from build123d import *

# Parameters (mm, degrees)
SKETCH1_W           = 9
SKETCH1_H           = 10
BOSS_EXTRUDE1_DEPTH = 3
SKETCH2_W           = 3
SKETCH2_H           = 10
BOSS_EXTRUDE2_DEPTH = 9
SKETCH3_W           = 10
SKETCH3_H           = 3
BOSS_EXTRUDE3_DEPTH = 17
SKETCH4_W           = 3
SKETCH4_H           = 10
BOSS_EXTRUDE4_DEPTH = 10
SKETCH5_W           = 10
SKETCH5_H           = 3
BOSS_EXTRUDE5_DEPTH = 6
CUT_EXTRUDE1_DEPTH  = 6


with BuildPart() as part:
    # Sketch1 → Boss-Extrude1 (new body)
    with BuildSketch(Plane(origin=(0, 0, 0), x_dir=(1, 0, 0), z_dir=(0, 1, 0))):
        with Locations((4.5, 5)):
            Rectangle(SKETCH1_W, SKETCH1_H)
    extrude(amount=BOSS_EXTRUDE1_DEPTH)

    # Sketch2 → Boss-Extrude2 (add)
    with BuildSketch(Plane(origin=(0, 3, 0), x_dir=(1, 0, 0), z_dir=(0, 1, 0))):
        with Locations((7.5, 5)):
            Rectangle(SKETCH2_W, SKETCH2_H)
    extrude(amount=BOSS_EXTRUDE2_DEPTH)

    # Sketch3 → Boss-Extrude3 (add)
    with BuildSketch(Plane(origin=(9, 0, 0), x_dir=(0, 0, -1), z_dir=(1, 0, 0))):
        with Locations((5, 10.5)):
            Rectangle(SKETCH3_W, SKETCH3_H)
    extrude(amount=BOSS_EXTRUDE3_DEPTH)

    # Sketch4 → Boss-Extrude4 (add)
    with BuildSketch(Plane.XZ.offset(-9)):
        with Locations((24.5, -5)):
            Rectangle(SKETCH4_W, SKETCH4_H)
    extrude(amount=BOSS_EXTRUDE4_DEPTH)

    # Sketch5 → Boss-Extrude5 (add)
    with BuildSketch(Plane(origin=(26, 0, 0), x_dir=(0, 0, -1), z_dir=(1, 0, 0))):
        with Locations((5, 0.5)):
            Rectangle(SKETCH5_W, SKETCH5_H)
    extrude(amount=BOSS_EXTRUDE5_DEPTH)

    # Sketch6 → Cut-Extrude1 (cut)
    with BuildSketch(Plane(origin=(0, 3, 0), x_dir=(1, 0, 0), z_dir=(0, 1, 0))):
        with BuildLine():
            ThreePointArc((4.351556364, 5), (3.912216535, 6.060660172), (2.851556364, 6.5))
            Line((2.851556364, 6.5), (2.851556364, 5))
            Line((2.851556364, 5), (4.351556364, 5))
        make_face()
        with BuildLine():
            Line((2.851556364, 5), (2.851556364, 6.5))
            ThreePointArc((2.851556364, 6.5), (1.790896192, 6.060660172), (1.351556364, 5))
            Line((1.351556364, 5), (2.851556364, 5))
        make_face()
        with BuildLine():
            Line((4.351556364, 5), (2.851556364, 5))
            Line((2.851556364, 5), (2.851556364, 3.5))
            ThreePointArc((2.851556364, 3.5), (3.912216535, 3.939339828), (4.351556364, 5))
        make_face()
        with BuildLine():
            Line((2.851556364, 3.5), (2.851556364, 5))
            Line((2.851556364, 5), (1.351556364, 5))
            ThreePointArc((1.351556364, 5), (1.790896192, 3.939339828), (2.851556364, 3.5))
        make_face()
        with BuildLine():
            ThreePointArc((30.491456548, 5), (30.002546741, 5.955884174), (29, 6.340133291))
            Line((29, 6.340133291), (29, 5))
            Line((29, 5), (30.491456548, 5))
        make_face()
        with BuildLine():
            Line((29, 5), (29, 6.340133291))
            ThreePointArc((29, 6.340133291), (27.997453259, 5.955884174), (27.508543452, 5))
            Line((27.508543452, 5), (29, 5))
        make_face()
        with BuildLine():
            Line((30.491456548, 5), (29, 5))
            Line((29, 5), (29, 3.340133291))
            ThreePointArc((29, 3.340133291), (30.060660172, 3.779473119), (30.5, 4.840133291))
            ThreePointArc((30.5, 4.840133291), (30.497862614, 4.920180707), (30.491456548, 5))
        make_face()
        with BuildLine():
            Line((29, 3.340133291), (29, 5))
            Line((29, 5), (27.508543452, 5))
            ThreePointArc((27.508543452, 5), (27.884249118, 3.83758655), (29, 3.340133291))
        make_face()
    extrude(amount=-CUT_EXTRUDE1_DEPTH, mode=Mode.SUBTRACT)


solid = part.part
Model file for the job. Use its own axes, mm. A direction names the side the tool comes from. Round coordinates to 2 decimals unless told otherwise and drop trailing zeros. Loops run counter-clockwise (first coordinate to the right, second up) from the corner with the lowest first, then second, coordinate; pieces in that order, holes last. Notation, with made-up numbers: (89.25, 17) -> (114.25, 17) arc R20 ccw to (114.25, 23) -> close; hole circle Ø10 at (-27, 29). An arc over 180 degrees is marked (long way). Answer as CSV lines item,"result". Start each with the question number.
1) Slice it at D-D (x = 28.5). List the corners of the cut face in (y, z).
2) Mould opens along X. For faces 4 (the face through (9, 4, -5)), 5 (the face through (14.7, 9.3, -10)), 6 (the face through (26, 7, -5)) say: +X half, -X half, draft (parallel to the pull), parting line (faces both ways), or undercut.
3) Slice it at A-A (y = 0.5). List the corners of the cut face in (x, z), plus the area to 3 significant figures.
4) Slice it at B-B (y = 8.5). List the corners of the cut face in (x, z).
5) Tool access for faces 1 (the face through (30.3, 2, -6)), 2 (the face through (5, 0, -5)), 3 (the face through (16, 9, -5)): list every direction of +Z, -Z, +X, -X, +Y, -Y with a clear straight run to the whole face (end or side of a thin tool).
6) Probe line 1 along X through (y, z) = (0.5, -2); line 2 along X through (y, z) = (6.25, -7.75); line 3 along X through (y, z) = (9.5, -9.5). List the from-to ranges inside material, lowest first.
7) Slice it at C-C (z = -4.5). List the corners of the cut face in (x, y), plus the area to 3 significant figures.
8) Pin check, flat tips, straight feed: P1, Ø3, axis at x = 2, z = -6.5, coming from the +Y side; P2, Ø5, axis at x = 17, z = -6, coming from the -Y side; P3, Ø1.8, axis at x = 30, z = -6.5, coming from the +Y side. Stop position of each tip, or through.
Filled in:
1,outline,"(-1, -10) -> (2, -10) -> (2, -6.25) -> (-1, -6.25) -> close; (-1, -3.43) -> (2, -3.43) -> (2, 0) -> (-1, 0) -> close"
2,face 4,"undercut"
2,face 5,"draft"
2,face 6,"+X half"
3,outline,"(0, -10) -> (9, -10) -> (9, 0) -> (0, 0) -> close; (23, -10) -> (32, -10) -> (32, 0) -> (23, 0) -> close; hole circle Ø3 at (2.85, -5); hole circle Ø3 at (29, -4.84)"
3,area,"166 mm2"
4,outline,"(6, -10) -> (9, -10) -> (9, 0) -> (6, 0) -> close; (23, -10) -> (26, -10) -> (26, 0) -> (23, 0) -> close"
5,face 1,"+Z, -Z, +X, +Y"
5,face 2,"+Z, -Z, -X, -Y"
5,face 3,"+Z, -Z, -Y"
6,line 1,"x = 0 to 9, 23 to 32"
6,line 2,"x = 6 to 9, 23 to 26"
6,line 3,"x = 6 to 26"
7,outline,"(0, 0) -> (1.44, 0) -> (1.44, 3) -> (0, 3) -> close; (4.27, 0) -> (9, 0) -> (9, 9) -> (23, 9) -> (23, -1) -> (27.54, -1) -> (27.54, 2) -> (26, 2) -> (26, 12) -> (6, 12) -> (6, 3) -> (4.27, 3) -> close; (30.46, -1) -> (32, -1) -> (32, 2) -> (30.46, 2) -> close"
7,area,"136 mm2"
8,P1,"stops at y = 3"
8,P2,"stops at y = 9"
8,P3,"stops at y = 2"
